Here's how the part is built. I have some questions about the finished solid (model axes, mm). A direction names the side the tool comes from. Round coordinates to 2 decimals unless told otherwise and drop trailing zeros. Loops run counter-clockwise (first coordinate to the right, second up) from the corner with the lowest first, then second, coordinate; pieces in that order, holes last. Notation, with made-up numbers: M 72,-13.75 L 123,-13.75 A26 ccw 123,15.25 Z; hole C 59.5,-11 d5. An arc over 180 degrees is marked long. Answer as a JSON object with one key per item and string values.
from build123d import *

# Parameters (mm, degrees)
PAD001_DEPTH    = 5
POCKET003_DEPTH = 2.501
PAD002_DEPTH    = 15


with BuildPart() as part:
    # Sketch005 → Pad001 (new body)
    with BuildSketch(Plane.XY.offset(8.5)):
        with BuildLine():
            ThreePointArc((0, -7.5), (7.5, 0), (0, 7.5))
            Line((0, 7.5), (-40, 7.5))
            Line((-40, 7.5), (-40, 3.25))
            Line((0, 3.25), (-40, 3.25))
            ThreePointArc((0, -3.25), (3.25, 0), (0, 3.25))
            Line((0, -3.25), (-40, -3.25))
            Line((-40, -3.25), (-40, -7.5))
            Line((0, -7.5), (-40, -7.5))
        make_face()
    extrude(amount=PAD001_DEPTH)

    # Sketch006 → Pocket003 (cut, through all)
    with BuildSketch(Plane.XY.offset(11)):
        with BuildLine():
            ThreePointArc((0, -5.5), (5.5, 0), (0, 5.5))
            Line((0, 5.5), (-40, 5.5))
            ThreePointArc((-40, 5.5), (-45.5, 0), (-40, -5.5))
            Line((0, -5.5), (-40, -5.5))
        make_face()
    extrude(amount=POCKET003_DEPTH, mode=Mode.SUBTRACT)

    # Sketch007 → Pad002 (join)
    with BuildSketch(Plane.XZ.offset(7.5)):
        Polygon((-40, 13.5), (-47.2, 13.5), (-48, 12.7), (-48, 11.9), (-41.875, 11.9), (-41.875, 10.1), (-48, 10.1), (-48, 9.3), (-47.2, 8.5), (-40, 8.5), align=None)
    extrude(amount=-PAD002_DEPTH)


solid = part.part
Item 1: I want a section at C-C, the plane y = -3.75. Please give me the cut outline in (x, z) (3 decimals).
Resolved:
{"outline": "M -48,9.3 L -47.2,8.5 L 6.495,8.5 L 6.495,13.5 L 4.023,13.5 L 4.023,11 L -40,11 L -40,13.5 L -47.2,13.5 L -48,12.7 L -48,11.9 L -41.875,11.9 L -41.875,10.1 L -48,10.1 Z"}
Item 2: If we mould it in two halves opening along X, with no side actions, what happens to faces 1 (the face through (5.5, -0.1, 12.2)), 2 (the face through (-41.875, 0, 11)), 3 (the face through (-24, -6, 13.5))? For each: pulls with the +X half, pulls with the -X half, needs draft (parallel to the pull), parting line crosses it, or undercut.
Resolved:
{"face 1": "undercut", "face 2": "pulls with the -X half", "face 3": "needs draft"}
Item 3: I want a section at A-A, the plane x = -18.5. Please give me the cut outline in (y, z), then the cut area to 4 significant figures.
Resolved:
{"outline": "M -7.5,8.5 L -3.25,8.5 L -3.25,11 L -5.5,11 L -5.5,13.5 L -7.5,13.5 Z; M 3.25,8.5 L 7.5,8.5 L 7.5,13.5 L 5.5,13.5 L 5.5,11 L 3.25,11 Z", "area": "31.25 mm²"}
Item 4: Please list where these lines run through material, in increasing order: probe 1 along Y at (x, z) = (-26.5, 13.1); probe 2 along Y at (x, z) = (-6, 9.3); probe 3 along X at (y, z) = (3, 10.7) (3 decimals). Write a range as from..to.
Resolved:
{"probe 1": "-7.5..-5.5, 5.5..7.5", "probe 2": "-7.5..-3.25, 3.25..7.5", "probe 3": "-41.875..-40, 1.25..6.874"}
Item 5: I want a section at D-D, the plane y = 6.5. Please give me the cut outline in (x, z) (3 decimals).
Resolved:
{"outline": "M -48,9.3 L -47.2,8.5 L 3.742,8.5 L 3.742,13.5 L -47.2,13.5 L -48,12.7 L -48,11.9 L -41.875,11.9 L -41.875,10.1 L -48,10.1 Z"}
Item 6: I want a section at B-B, the plane y = 0. Please give me the cut outline in (x, z) (3 decimals), then the cut area to 3 significant figures.
Resolved:
{"outline": "M -48,9.3 L -47.2,8.5 L -40,8.5 L -40,13.5 L -47.2,13.5 L -48,12.7 L -48,11.9 L -41.875,11.9 L -41.875,10.1 L -48,10.1 Z; M 3.25,8.5 L 7.5,8.5 L 7.5,13.5 L 5.5,13.5 L 5.5,11 L 3.25,11 Z", "area": "44.0 mm²"}
Item 7: On a 3-axis mill with a long thin cutter (end or side, diameter ignored), from which of +Z, -Z, +X, -X, +Y, -Y can I reach the whole of each face in a straight line? I mean faces 4 (the face through (-20, 3.25, 10)), 5 (the face through (-24, -7.5, 11)), 6 (the face through (-40, 0, 12)), 7 (the face through (7.5, -0.16, 10.96)), 8 (the face through (-45, 0, 10.1)). Say none if no direction works.
Resolved:
{"face 4": "+Z, -Z", "face 5": "+Z, -Z, +X, -X, -Y", "face 6": "+Z", "face 7": "+Z, -Z, +X", "face 8": "-X, +Y, -Y"}
Item 8: I'm going to push flat-ended pins straight in: pin 1 Ø1.5 at (y, z) = (-1, 11.5) entering from +X; pin 2 Ø1.4 at (y, z) = (3.5, 11) entering from -X (3 decimals). Where does each tip first touch, or does it pass through?
Resolved:
{"pin 1": "x = 7.5", "pin 2": "x = -41.875"}
